Work out the finished part from the listing and answer in its coordinate system (mm). A direction names the side the tool comes from. Give positions to 0.01 mm unless a question says otherwise; leave off trailing zeros. Write each loop counter-clockwise with the first axis right and the second up, starting at its lowest first coordinate (ties: lowest second). Pieces come first, ordered by that corner, then holes. Notation, with made-up numbers: (-9.75, 85) - (6.25, 85) arc R21 ccw to (6.25, 97) - close; hole circle Ø9 at (-18, -37). An arc over 180 degrees is marked (long way). Write each question's results on one line, items separated by ' | '. Start each with the question number.
from build123d import *

# Parameters (mm, degrees)
F0_R     = 1.651
F1_DEPTH = 25.4


with BuildPart() as f1:
    # F0 (on Top) → F1 (new body)
    with BuildSketch(Plane.XY):
        with BuildLine():
            Line((5.9660125897, 0), (0, 0))
            Line((0, 0), (0, -50.8))
            Line((0, -50.8), (5.9660125897, -50.8))
            ThreePointArc((5.9660125897, -50.8), (26.8404151011, -54.2874891517), (45.4474833472, -64.3711527752))
            ThreePointArc((45.4474833472, -64.3711527752), (67.7366219489, -78.6995467545), (92.2477625944, -88.7649606997))
            Line((92.2477625944, -88.7649606997), (96.1756392809, -85.285625491))
            ThreePointArc((96.1756392809, -85.285625491), (96.6297262922, -84.9647009914), (97.1427657695, -84.7502760791))
            Line((97.1427657695, -84.7502760791), (97.1427657695, -70.3371887059))
            ThreePointArc((97.1427657695, -70.3371887059), (77.2725114585, -62.1844747684), (59.0602220587, -50.8))
            Line((59.0602220587, -50.8), (59.0253094804, 0))
            ThreePointArc((59.0253094804, 0), (77.2534891322, 11.396761217), (97.1427657695, 19.555766947))
            Line((97.1427657695, 19.555766947), (97.1427657695, 33.9761360632))
            ThreePointArc((97.1427657695, 33.9761360632), (96.6371725478, 34.190077646), (96.1893595345, 34.5076607246))
            Line((96.1893595345, 34.5076607246), (92.2622799467, 37.987895583))
            ThreePointArc((92.2622799467, 37.987895583), (67.7168934482, 27.9114522536), (45.3996037793, 13.5605188218))
            ThreePointArc((45.3996037793, 13.5605188218), (26.8160472709, 3.4848333701), (5.9660125897, 0))
        make_face()
        with Locations((17.272, -25.4)):
            Circle(F0_R, mode=Mode.SUBTRACT)
        with Locations((27.178, -25.4)):
            Circle(F0_R, mode=Mode.SUBTRACT)
        with BuildLine():
            Line((173.3427657695, 33.9685711851), (173.3427657695, 19.5447874489))
            ThreePointArc((173.3427657695, 19.5447874489), (193.2134106927, 11.3884070061), (211.4253094804, 0))
            ThreePointArc((211.4253094804, 0), (224.7603094804, 1.905), (222.8553094804, 15.24))
            ThreePointArc((222.8553094804, 15.24), (201.5199367106, 28.5369467154), (178.2203126555, 37.9780505738))
            Line((178.2203126555, 37.9780505738), (174.292435969, 34.4987153651))
            ThreePointArc((174.292435969, 34.4987153651), (173.8463095868, 34.1822161077), (173.3427657695, 33.9685711851))
        make_face()
        with BuildLine():
            ThreePointArc((211.4253094804, -50.8), (193.2130200806, -62.1844747684), (173.3427657695, -70.3371887059))
            Line((173.3427657695, -70.3371887059), (173.3427657695, -84.7683622579))
            ThreePointArc((173.3427657695, -84.7683622579), (173.8388638616, -84.9814448856), (174.2787157154, -85.2945708506))
            Line((174.2787157154, -85.2945708506), (178.2057953033, -88.7748057089))
            ThreePointArc((178.2057953033, -88.7748057089), (201.5113077809, -79.337141934), (222.852691037, -66.0419634811))
            ThreePointArc((222.852691037, -66.0419634811), (224.7599819992, -52.7072909622), (211.4253094804, -50.8))
        make_face()
        with BuildLine():
            ThreePointArc((128.892021211, 44.312617548), (115.3953137669, 43.0975250998), (102.0693249913, 40.6367153465))
            Line((102.0693249913, 40.6367153465), (100.2677893758, 35.5592610119))
            ThreePointArc((100.2677893758, 35.5592610119), (99.5924476221, 34.538163122), (98.5179053993, 33.9515743424))
            Line((98.5179053993, 33.9515743424), (101.8073036013, 20.9244338206))
            ThreePointArc((101.8073036013, 20.9244338206), (118.374331468, 24.2771009359), (135.2398551386, 25.399999167))
            Line((135.2398551386, 25.399999167), (135.2414022457, 38.9079894532))
            ThreePointArc((135.2414022457, 38.9079894532), (133.6409701921, 39.2606320138), (132.3367275841, 40.2529478676))
            Line((132.3367275841, 40.2529478676), (128.892021211, 44.312617548))
        make_face()
        with BuildLine():
            ThreePointArc((98.5179053993, 33.9515743424), (97.8286414895, 33.8690077361), (97.1427657695, 33.9761360632))
            Line((97.1427657695, 33.9761360632), (97.1427657695, 19.555766947))
            ThreePointArc((97.1427657695, 19.555766947), (99.468485514, 20.2624205399), (101.8073036013, 20.9244338206))
            Line((101.8073036013, 20.9244338206), (98.5179053993, 33.9515743424))
        make_face()
        with BuildLine():
            Line((135.2414022457, 38.9079894532), (135.2398551386, 25.399999167))
            ThreePointArc((135.2398551386, 25.399999167), (154.5147695349, 23.9265578705), (173.3427657695, 19.5447874489))
            Line((173.3427657695, 19.5447874489), (173.3427657695, 33.9685711851))
            ThreePointArc((173.3427657695, 33.9685711851), (171.46164391, 34.1335607927), (170.2142471201, 35.5512498522))
            Line((170.2142471201, 35.5512498522), (168.4138746214, 40.6291167233))
            ThreePointArc((168.4138746214, 40.6291167233), (155.088449882, 43.092978936), (141.5920211277, 44.3111629821))
            Line((141.5920211277, 44.3111629821), (138.1463849147, 40.2522824716))
            ThreePointArc((138.1463849147, 40.2522824716), (136.8419150357, 39.2602654008), (135.2414022457, 38.9079894532))
        make_face()
        with BuildLine():
            ThreePointArc((173.3427657695, -70.3371887059), (154.5088049536, -74.7170648066), (135.2282201113, -76.186909293))
            Line((135.2282201113, -76.186909293), (135.2266730042, -89.6948995791))
            ThreePointArc((135.2266730042, -89.6948995791), (136.8271050578, -90.0475421398), (138.1313476658, -91.0398579935))
            Line((138.1313476658, -91.0398579935), (141.5760540389, -95.0995276739))
            ThreePointArc((141.5760540389, -95.0995276739), (155.072761483, -93.8844352257), (168.3987502586, -91.4236254724))
            Line((168.3987502586, -91.4236254724), (170.2002858741, -86.3461711378))
            ThreePointArc((170.2002858741, -86.3461711378), (171.4543564481, -84.9255689093), (173.3427657695, -84.7683622579))
            Line((173.3427657695, -84.7683622579), (173.3427657695, -70.3371887059))
        make_face()
        with BuildLine():
            Line((100.2538281298, -86.3381599782), (102.0542006285, -91.4160268492))
            ThreePointArc((102.0542006285, -91.4160268492), (115.3796253679, -93.879889062), (128.8760541222, -95.0980731081))
            Line((128.8760541222, -95.0980731081), (132.3216903352, -91.0391925976))
            ThreePointArc((132.3216903352, -91.0391925976), (133.6261602142, -90.0471755268), (135.2266730042, -89.6948995791))
            Line((135.2266730042, -89.6948995791), (135.2282201113, -76.186909293))
            ThreePointArc((135.2282201113, -76.186909293), (115.962349399, -74.714857391), (97.1427657695, -70.3371887059))
            Line((97.1427657695, -70.3371887059), (97.1427657695, -84.7502760791))
            ThreePointArc((97.1427657695, -84.7502760791), (99.0145511059, -84.9245969075), (100.2538281298, -86.3381599782))
        make_face()
    extrude(amount=F1_DEPTH)


solid = f1.part
Q1. A cutting plane is placed at A-A, the plane x = 73.5. Write down the section's boundary in (y, z).
Q2. Consider L1, parallel to Y at x = 172, z = 7.5; L2, parallel to X at y = -43.5, z = 24.75; L3, parallel to X at y = 13.5, z = 10.75. Determine where each line is inside the solid, lowest interval first.
Q3. A cutting plane is placed at C-C, the plane z = 22. Give the number of separate pieces and of enclosed holes in the cut face, and give its area (3 significant figures).
Q4. A cutting plane is placed at D-D, the plane y = -18. Write down the section's boundary in (x, z).
Q5. The mould has two halves that part along X. Classify faces 4 (the flat face through (0, -25, 13)), 5 (the flat face through (139.893, 42.31, 12.522)), 6 (the cylindrical face through (201.197, -79.497, 12.522)), 7 (the flat face through (88, 21, 0)): pulls with the +X half, pulls with the -X half, needs draft (parallel to the pull), parting line crosses it, or undercut.
Q6. Given pin 1 (4 mm diameter, centred on x = 17.272, y = -25.4, fed in from +Z); pin 2 (3 mm diameter, centred on x = 3.5, z = 7, fed in from -Y); pin 3 (3 mm diameter, centred on x = 27.178, y = -25.4, fed in from +Z); pin 4 (1.8 mm diameter, centred on x = 2, z = 12, fed in from +Y), each flat-ended and moving along its own axis, determine where each tip first touches the part or whether it passes through.
Q7. A cutting plane is placed at B-B, the plane y = -55.5. Write down the section's boundary in (x, z), and give its area (3 significant figures).
Q8. A tool of negligible diameter and unlimited length cuts with its end or side. For faces 1 (the flat face through (130.6, 42.3, 12.5)), 2 (the flat face through (169.287, -88.92, 12.522)), 3 (the cylindrical face through (224.6, 1.7, 12.5)), from which of +Z, -Z, +X, -X, +Y, -Y can it reach the whole face along a straight path? Write none if from no direction.
Result:
1) outline: (-81.54, 0) - (-60.17, 0) - (-60.17, 25.4) - (-81.54, 25.4) - close; (9.39, 0) - (30.77, 0) - (30.77, 25.4) - (9.39, 25.4) - close
2) L1: y = -84.73 to -70.75, 19.96 to 33.93 | L2: x = 0 to 59.06 | L3: x = 45.32 to 81.55, 188.9 to 224.63
3) separate pieces: 1 | enclosed holes: 2 | area: 10,300 mm2
4) outline: (0, 0) - (59.04, 0) - (59.04, 25.4) - (0, 25.4) - close
5) face 4: pulls with the -X half | face 5: undercut | face 6: pulls with the +X half | face 7: needs draft
6) pin 1: stops at z = 25.4 | pin 2: stops at y = -50.8 | pin 3: passes through | pin 4: stops at y = 0
7) outline: (30.08, 0) - (65.77, 0) - (65.77, 25.4) - (30.08, 25.4) - close; (204.72, 0) - (226.21, 0) - (226.21, 25.4) - (204.72, 25.4) - close | area: 1,450 mm2
8) face 1: +Z, -Z, +Y | face 2: +Z, -Z, -Y | face 3: +Z, -Z
